```python
from build123d import *

# Parameters (mm, degrees)
SKETCH1_R           = 5.5
BOSS_EXTRUDE1_DEPTH = 15
SKETCH2_R           = 18
SKETCH2_R_2         = 5.5
BOSS_EXTRUDE3_DEPTH = 3
SKETCH3_R           = 12.86
SKETCH3_R_2         = 9.86
BOSS_EXTRUDE4_DEPTH = 10


with BuildPart() as part:
    # Sketch1 → Boss-Extrude1 (new body)
    with BuildSketch(Plane(origin=(0, 0, 0), x_dir=(1, 0, 0), z_dir=(0, 1, 0))):
        with Locations(Location((2.5, 2.5, 0), (0, 0, 270))):
            Circle(SKETCH1_R)
        with BuildLine():
            Line((4, 0.5), (1, 0.5))
            ThreePointArc((1, 0.5), (2.5, 5), (4, 0.5))
        make_face(mode=Mode.SUBTRACT)
    extrude(amount=BOSS_EXTRUDE1_DEPTH)

    # Sketch2 → Boss-Extrude3 (add)
    with BuildSketch(Plane(origin=(0, 15, 0), x_dir=(1, 0, 0), z_dir=(0, 1, 0))):
        with Locations((2.5, 2.5)):
            Circle(SKETCH2_R)
        with Locations(Location((2.5, 2.5, 0), (0, 0, 270))):
            Circle(SKETCH2_R_2, mode=Mode.SUBTRACT)
        with Locations(Location((2.5, 2.5, 0), (0, 0, 270))):
            Circle(SKETCH2_R_2)
        with BuildLine():
            Line((4, 0.5), (1, 0.5))
            ThreePointArc((1, 0.5), (2.5, 5), (4, 0.5))
        make_face(mode=Mode.SUBTRACT)
        with BuildLine():
            ThreePointArc((20.5, 2.5), (2.5, -15.5), (-15.5, 2.5))
            Line((-15.5, 2.5), (-15.5, -67.5))
            Line((-15.5, -67.5), (2.5, -77.5))
            Line((2.5, -77.5), (20.5, -67.5))
            Line((20.5, -67.5), (20.5, 2.5))
        make_face()
    extrude(amount=BOSS_EXTRUDE3_DEPTH)

    # Sketch3 → Boss-Extrude4 (add)
    with BuildSketch(Plane.XZ.offset(-15)):
        with Locations(Location((2.5, 52.5, 0), (0, 0, 90))):
            Circle(SKETCH3_R)
        with Locations(Location((2.5, 52.5, 0), (0, 0, 270))):
            Circle(SKETCH3_R_2, mode=Mode.SUBTRACT)
    extrude(amount=BOSS_EXTRUDE4_DEPTH)


solid = part.part
```
Part model, mm, in its own coordinate system. A direction names the side the tool comes from. Round coordinates to 2 decimals unless told otherwise and drop trailing zeros. Write each loop counter-clockwise with the first axis right and the second up, starting at its lowest first coordinate (ties: lowest second). Pieces come first, ordered by that corner, then holes.
Item 1: Drop flat-ended pins along their axis: pin 1 Ø3.5 at (x, y) = (2, 10) entering from -Z; pin 2 Ø16 at (x, z) = (3.5, 50.5) entering from -Y; pin 3 Ø4 at (y, z) = (9.5, 47) entering from +X. Give the stop position or say it passes through.
Results:
pin 1: stops at z = -8
pin 2: stops at y = 5
pin 3: stops at x = 14.87
Item 2: Cut at D-D, the plane x = -4. Give the cut face in (y, z), plus the area to 3 significant figures.
Results:
outline: (5, 41.4) - (15, 41.4) - (15, -19.29) - (18, -19.29) - (18, 73.89) - (15, 73.89) - (15, 63.6) - (5, 63.6) - (5, 59.91) - (15, 59.91) - (15, 45.09) - (5, 45.09) - close
area: 353 mm2
Item 3: Cut at B-B, the plane z = 52.5. Give the cut face in (x, y), plus the area to 3 significant figures.
Results:
outline: (-15.5, 15) - (-10.36, 15) - (-10.36, 5) - (-7.36, 5) - (-7.36, 15) - (12.36, 15) - (12.36, 5) - (15.36, 5) - (15.36, 15) - (20.5, 15) - (20.5, 18) - (-15.5, 18) - close
area: 168 mm2
Item 4: Probe L1, parallel to X at y = 10, z = 52.5; L2, parallel to X at y = 14.25, z = -2.5; L3, parallel to Y at x = -11, z = -7. List the from-to ranges inside material, lowest first.
Results:
L1: x = -10.36 to -7.36, 12.36 to 15.36
L2: x = -3 to 0, 5 to 8
L3: y = 15 to 18
Item 5: Cut at A-A, the plane y = 7. Give the cut face in (x, z).
Results:
outline: circle Ø25.72 at (2.5, 52.5); circle Ø11 at (2.5, -2.5); hole circle Ø19.72 at (2.5, 52.5); hole (1, -0.5) arc R2.5 ccw (long way) to (4, -0.5) - close
Item 6: Two-plate mould, pull along Z, no slides. Class faces 1 (the flat face through (3, 9, -0.5)), 2 (the flat face through (2, 15, 28)), 3 (the flat face through (11.37, 16.48, 72.57)), 4 (the flat face through (10.1, 5, 59.1)): +Z half, -Z half, draft (parallel to the pull), parting line (faces both ways), or undercut.
Results:
face 1: undercut
face 2: undercut
face 3: +Z half
face 4: draft
Item 7: Which spindle directions (+Z, -Z, +X, -X, +Y, -Y) get a long thin tool onto all of the face, cutting with end or side? Do faces 5 (the flat face through (2, 15, 52)), 6 (the flat face through (20.5, 16, 33)). Say none if no direction does.
Results:
face 5: -Y
face 6: +Z, -Z, +X, +Y, -Y
Item 8: Cut at C-C, the plane y = 1.5. Give the cut face in (x, z), plus the area to 3 significant figures.
Results:
outline: circle Ø11 at (2.5, -2.5); hole (1, -0.5) arc R2.5 ccw (long way) to (4, -0.5) - close
area: 76.4 mm2
